Verification items for the finished model (mm, model axes). A direction names the side the tool comes from. Round coordinates to 2 decimals unless told otherwise and drop trailing zeros. Loops run counter-clockwise (first coordinate to the right, second up) from the corner with the lowest first, then second, coordinate; pieces in that order, holes last. Notation, with made-up numbers: M 3,63 L 58,63 A13 ccw 58,75 Z; hole C 65,-13 d1. An arc over 180 degrees is marked long. Write item = value, one per line. Start each with the question number.
from build123d import *

# Parameters (mm, degrees)
SKETCH1_R                      = 4.7625
BOSS_EXTRUDE1_DEPTH            = 6.35
F_3_16_0_1875_DIAMETER_HOLE1_D = 4.7625
F_6_32_TAPPED_HOLE1_D          = 2.7051
F_6_32_TAPPED_HOLE1_DEPTH      = 22.352
F_6_32_TAPPED_HOLE1_TIP        = 0.81269403
F_6_CLEARANCE_HOLE1_D          = 3.7973
F_6_CLEARANCE_HOLE1_DEPTH      = 6.35
F_6_CLEARANCE_HOLE1_TIP        = 1.140824014


with BuildPart() as part:
    # Sketch1 → Boss-Extrude1 (new body)
    with BuildSketch(Plane(origin=(0, 0, 0), x_dir=(1, 0, 0), z_dir=(0, 1, 0))):
        with BuildLine():
            Line((6.35, 24), (6.35, 0))
            ThreePointArc((6.35, 0), (0, -6.35), (-6.35, 0))
            Line((-6.35, 0), (-6.35, 24))
            ThreePointArc((-6.35, 24), (0, 30.35), (6.35, 24))
        make_face()
        with Locations((0, 24)):
            Circle(SKETCH1_R, mode=Mode.SUBTRACT)
    extrude(amount=BOSS_EXTRUDE1_DEPTH)

    # 3/16 (0.1875) Diameter Hole1 (through all)
    with Locations(Plane(origin=(0, 6.35, 0), x_dir=(1, 0, 0), z_dir=(0, 1, 0))):
        with Locations((0, 0)):
            Hole(F_3_16_0_1875_DIAMETER_HOLE1_D / 2)

    # #6-32 Tapped Hole1
    with Locations(Plane(origin=(0, 0, -30.35), x_dir=(-1, 0, 0), z_dir=(0, 0, -1))):
        with Locations((0, 3.175)):
            Hole(F_6_32_TAPPED_HOLE1_D / 2, depth=F_6_32_TAPPED_HOLE1_DEPTH)
            with Locations((0, 0, -(F_6_32_TAPPED_HOLE1_DEPTH + F_6_32_TAPPED_HOLE1_TIP / 2))):  # 118° drill point
                Cone(0, F_6_32_TAPPED_HOLE1_D / 2, F_6_32_TAPPED_HOLE1_TIP, mode=Mode.SUBTRACT)

    # #6 Clearance Hole1
    with Locations(Plane(origin=(0, 0, -30.35), x_dir=(-1, 0, 0), z_dir=(0, 0, -1))):
        with Locations((0, 3.175)):
            Hole(F_6_CLEARANCE_HOLE1_D / 2, depth=F_6_CLEARANCE_HOLE1_DEPTH)
            with Locations((0, 0, -(F_6_CLEARANCE_HOLE1_DEPTH + F_6_CLEARANCE_HOLE1_TIP / 2))):  # 118° drill point
                Cone(0, F_6_CLEARANCE_HOLE1_D / 2, F_6_CLEARANCE_HOLE1_TIP, mode=Mode.SUBTRACT)


solid = part.part
1. Thickness scan on line 1 (Z direction, x = 0, y = 5.25); line 2 (Y direction, x = 0, z = -29.5); line 3 (Z direction, x = -1.75, y = 0.75). Record the ranges inside material, lowest first.
2. Section check B-B, the plane z = 1.5. Enter the section's corners in (x, y).
3. Tool access check on faces 5 (the cylindrical face through (1.81, 3.75, -29.35)), 6 (the cylindrical face through (1.89, 3.13, 1.45)). Record the directions out of +Z, -Z, +X, -X, +Y, -Y that give a thin tool (end or side, any length) a straight path to the whole face; none if there is none.
4. Section check C-C, the plane z = -9.5. Enter the section's corners in (x, y) (3 decimals).
5. Section check A-A, the plane y = 5.5. Give the number of separate pieces and of enclosed holes in the cut face, and give its area (3 significant figures).
6. Gauge pin test, flat ends, axial feed: P1, Ø6, axis at x = 0, z = 0, coming from the -Y side; P2, Ø2, axis at x = 3, y = 1, coming from the -Z side; P3, Ø1, axis at x = 3, y = 1.5, coming from the -Z side; P4, Ø2.5, axis at x = 0, y = 3.175, coming from the -Z side. Record the tip position at first contact, or that the pin passes through.
7. Mould release check, pull along X, two halves, no side actions. Record for faces 1 (the cylindrical face through (0.14, 3.13, 6.35)), 2 (the cylindrical face through (0.727, 4.315, -13.639)), 3 (the flat face through (0, 0, -8)), 4 (the flat face through (-6.35, 3, -12)): pulls with the +X half, pulls with the -X half, needs draft (parallel to the pull), parting line crosses it, or undercut.
Computed values:
q1.line_1 = -30.35 to -28.76, -19.24 to -2.38, 2.38 to 6.35
q1.line_2 = 0 to 1.28, 5.07 to 6.35
q1.line_3 = -30.1 to -28.43, -19.57 to -1.61, 1.61 to 6.1
q2.outline = M -6.17,0 L -1.85,0 L -1.85,6.35 L -6.17,6.35 Z; M 1.85,0 L 6.17,0 L 6.17,6.35 L 1.85,6.35 Z
q3.face_5 = -Z
q3.face_6 = +Y, -Y
q4.outline = M -6.35,0 L 6.35,0 L 6.35,6.35 L -6.35,6.35 Z; hole C 0,3.175 d2.705
q5.separate_pieces = 1
q5.enclosed_holes = 2
q5.area = 342 mm2
q6.P1 = 0
q6.P2 = -30.03
q6.P3 = -29.84
q6.P4 = -7.94
q7.face_1 = parting line crosses it
q7.face_2 = undercut
q7.face_3 = needs draft
q7.face_4 = pulls with the -X half
